Geometry check sheet. Reference: drawing and pictorial views, mm from the part's lowest x, y, z. Round coordinates to 2 decimals unless told otherwise and drop trailing zeros. Order: outer loops, then holes, each group sorted by start corner. A loop starts at its lowest first (then second) coordinate and runs counter-clockwise, first axis right, second up.
Q1. Depth check by flat-ended pin: P1, Ø6, axis at x = 5, y = 12.5, coming from the -Z side. Enter the tip coordinate at first touch or a pass-through.
Q2. Cross-section at A-A on y = 9. Record the cut outline in (x, z), then the cut area to 3 significant figures.
Q3. Mould release check, pull along Y, two halves, no side actions. Record for the marked faces 1, 2 and 3: +Y half, -Y half, draft (parallel to the pull), parting line (faces both ways), or undercut.
Q4. Cross-section at B-B on x = 5. Record the cut outline in (y, z), then the cut area to 3 significant figures.
Q5. Cross-section at C-C on z = 7.5. Record the cut outline in (x, y), then the cut area to 3 significant figures.
Q6. Scan lines: probe 1 along Y at (x, z) = (5, 4); probe 2 along Y at (x, z) = (5, 0.8); probe 3 along Z at (x, y) = (3.5, 12). Record each from-to range of solid material in increasing order.
Q7. Cross-section at D-D on x = 3. Record the cut outline in (y, z).
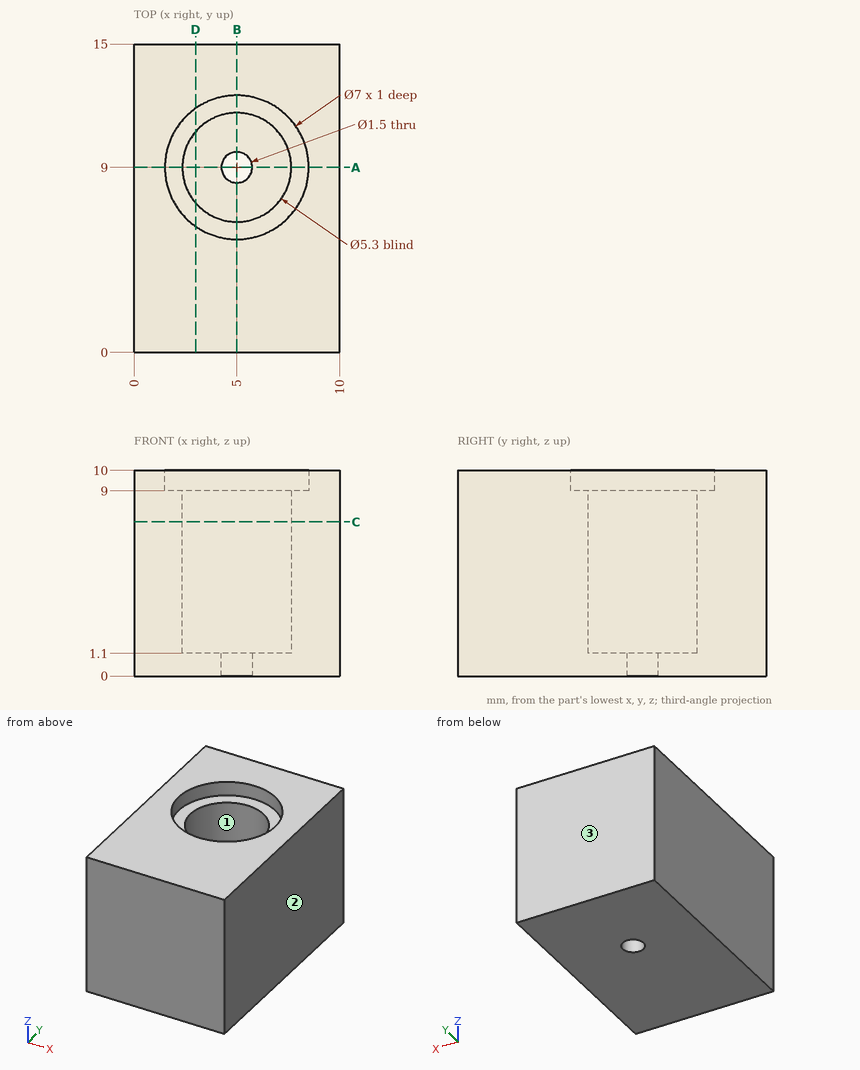
Results found:
1. P1: stops at z = 0
2. outline: (0, 0) - (4.25, 0) - (4.25, 1.1) - (2.35, 1.1) - (2.35, 9) - (1.5, 9) - (1.5, 10) - (0, 10) - close; (5.75, 0) - (10, 0) - (10, 10) - (8.5, 10) - (8.5, 9) - (7.65, 9) - (7.65, 1.1) - (5.75, 1.1) - close
2. area: 49.5 mm2
3. face 1: undercut
3. face 2: draft
3. face 3: +Y half
4. outline: (0, 0) - (8.25, 0) - (8.25, 1.1) - (6.35, 1.1) - (6.35, 9) - (5.5, 9) - (5.5, 10) - (0, 10) - close; (9.75, 0) - (15, 0) - (15, 10) - (12.5, 10) - (12.5, 9) - (11.65, 9) - (11.65, 1.1) - (9.75, 1.1) - close
4. area: 99.5 mm2
5. outline: (0, 0) - (10, 0) - (10, 15) - (0, 15) - close; hole circle Ø5.3 at (5, 9)
5. area: 128 mm2
6. probe 1: y = 0 to 6.35, 11.65 to 15
6. probe 2: y = 0 to 8.25, 9.75 to 15
6. probe 3: z = 0 to 9
7. outline: (0, 0) - (15, 0) - (15, 10) - (11.87, 10) - (11.87, 9) - (10.74, 9) - (10.74, 1.1) - (7.26, 1.1) - (7.26, 9) - (6.13, 9) - (6.13, 10) - (0, 10) - close
